Here's the drawing with two shaded views (mm, measured from the low corner). I have some questions. Round coordinates to 2 decimals unless told otherwise and drop trailing zeros. Loops run counter-clockwise (first coordinate to the right, second up) from the corner with the lowest first, then second, coordinate; pieces in that order, holes last. Notation, with made-up numbers: (34.5, 23) -> (81.5, 23) arc R21 cw to (81.5, 44) -> close; hole circle Ø1 at (67.5, 60.5). An arc over 180 degrees is marked (long way). Write item = value, one per line.
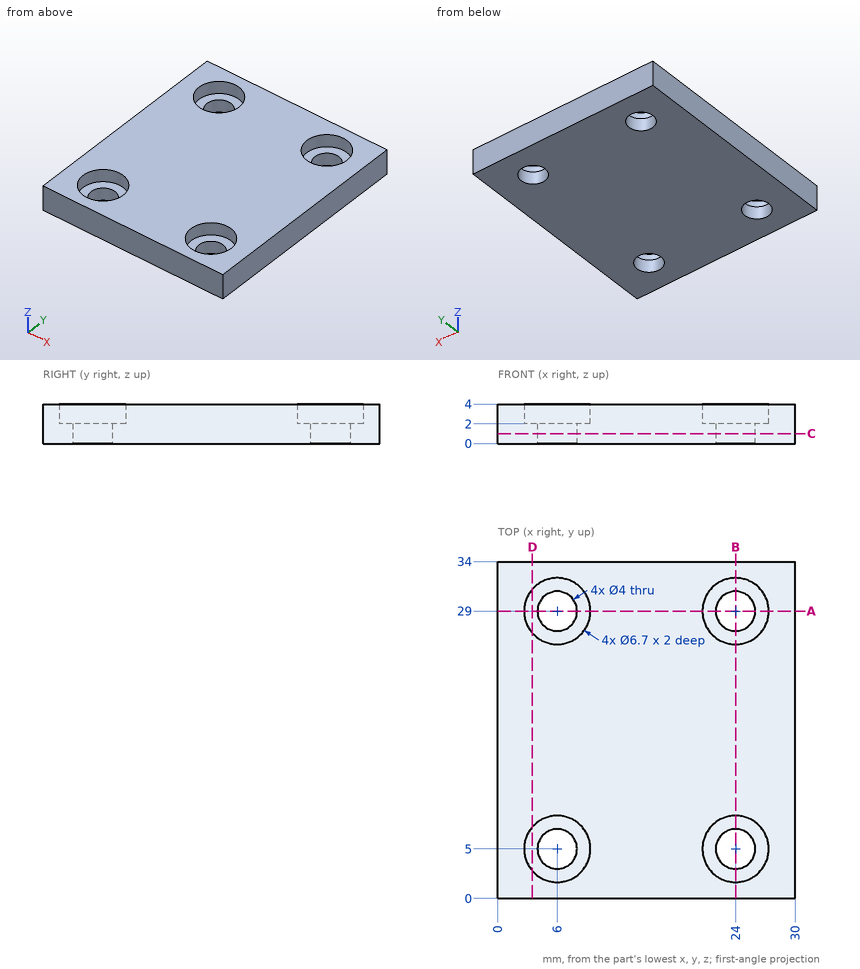
1. Suppose I cut it at C-C, the plane z = 1. List the corners of the cut face in (x, y) for me, and give its area (3 significant figures).
Entries:
outline = (0, 0) -> (30, 0) -> (30, 34) -> (0, 34) -> close; hole circle Ø4 at (6, 5); hole circle Ø4 at (6, 29); hole circle Ø4 at (24, 5); hole circle Ø4 at (24, 29)
area = 970 mm²
2. I'm going to push flat-ended pins straight in: pin 1 (2.5 mm diameter, centred on x = 24, y = 29, fed in from +Z); pin 2 (3.5 mm diameter, centred on x = 24.5, y = 5, fed in from +Z). Where does each tip first touch, or does it pass through?
Entries:
pin_1 = through
pin_2 = 2
3. I need wall thicknesses on line 1 (Y direction, x = 24, z = 2.55); line 2 (Y direction, x = 24, z = 0.6); line 3 (X direction, y = 4.5, z = 3.45). Which ranges of each line are inside material? Lowest first, please. Write a range as [from, to].
Entries:
line_1 = [0, 1.65], [8.35, 25.65], [32.35, 34]
line_2 = [0, 3], [7, 27], [31, 34]
line_3 = [0, 2.69], [9.31, 20.69], [27.31, 30]
4. Suppose I cut it at D-D, the plane x = 3.5. List the corners of the cut face in (y, z) for me.
Entries:
outline = (0, 0) -> (34, 0) -> (34, 4) -> (31.23, 4) -> (31.23, 2) -> (26.77, 2) -> (26.77, 4) -> (7.23, 4) -> (7.23, 2) -> (2.77, 2) -> (2.77, 4) -> (0, 4) -> close
5. Suppose I cut it at A-A, the plane y = 29. List the corners of the cut face in (x, z) for me.
Entries:
outline = (0, 0) -> (4, 0) -> (4, 2) -> (2.65, 2) -> (2.65, 4) -> (0, 4) -> close; (8, 0) -> (22, 0) -> (22, 2) -> (20.65, 2) -> (20.65, 4) -> (9.35, 4) -> (9.35, 2) -> (8, 2) -> close; (26, 0) -> (30, 0) -> (30, 4) -> (27.35, 4) -> (27.35, 2) -> (26, 2) -> close
6. Suppose I cut it at B-B, the plane x = 24. List the corners of the cut face in (y, z) for me, and give its area (3 significant figures).
Entries:
outline = (0, 0) -> (3, 0) -> (3, 2) -> (1.65, 2) -> (1.65, 4) -> (0, 4) -> close; (7, 0) -> (27, 0) -> (27, 2) -> (25.65, 2) -> (25.65, 4) -> (8.35, 4) -> (8.35, 2) -> (7, 2) -> close; (31, 0) -> (34, 0) -> (34, 4) -> (32.35, 4) -> (32.35, 2) -> (31, 2) -> close
area = 93.2 mm²
